Read the model definition and answer for the solid it produces. Units are mm, in the model's axes. Face numbers are marked on the shaded views. A direction names the side the tool comes from. Coordinates: 2 decimals unless noted, no trailing zeros. Loops run counter-clockwise (first coordinate to the right, second up) from the corner with the lowest first, then second, coordinate; pieces in that order, holes last. Notation, with made-up numbers: M -19.5,-22 L 11.5,-22 A10 ccw 11.5,-10 Z; hole C -8.75,13 d8. An arc over 180 degrees is marked long. Use one line per item in the form item = value. Start each with the question number.
1. A tool of negligible diameter and unlimited length cuts with its end or side. For the marked faces 5, 6, 7 and 8, from which of +Z, -Z, +X, -X, +Y, -Y can it reach the whole face along a straight path? Write none if from no direction.
2. Flat-ended cylindrical pins translate along their axes: pin 1 (3.5 mm diameter, centred on x = -19.5, y = -15, fed in from +Z); pin 2 (3.5 mm diameter, centred on x = 17.55, z = 4.4, fed in from +Y); pin 3 (3 mm diameter, centred on y = -28, z = 17.5, fed in from +X). Find the tip coordinate at first contact, or state that the pin passes through.
3. Find the intervals of material crossed by probe 1 along Z at (x, y) = (0, -4) (3 decimals); probe 2 along Z at (x, y) = (0, -25) (3 decimals); probe 3 along Z at (x, y) = (-14, -5), in increasing order. Write a range as [from, to].
4. The part is cut by section B-B (x = 0). Give the vertices of the cut face in (y, z) (3 decimals), plus the area to 3 significant figures.
5. The part is cut by section C-C (z = 3). Give the vertices of the cut face in (x, y).
6. For a pull along Z with two mould halves and no side action, classify the marked faces 1, 2, 3 and 4 as released by +Z, released by -Z, zero draft, split by the parting line, or undercut.
7. The part is cut by section A-A (y = -3). Give the number of separate pieces and of enclosed holes in the cut face, plus the area to 3 significant figures.
from build123d import *

# Parameters (mm, degrees)
F0_R     = 25.85
F0_R_2   = 4.9
F0_R_3   = 2.1
F1_DEPTH = 1.6
F0_R_4   = 27.45
F2_DEPTH = 10
F3_R     = 12.375
F4_DEPTH = 32.5
F6_DEPTH = 5


# Not quite as in the source:
# - ends of sketch curves that miss each other by under 0.0002 mm in the source are joined


with BuildPart() as f1:
    # F0 (on Front) → F1 (new body)
    with BuildSketch(Plane.XZ):
        Circle(F0_R)
        with Locations((0, -3.85)):
            Circle(F0_R_2, mode=Mode.SUBTRACT)
        with Locations((-17.55, 4.4)):
            Circle(F0_R_3, mode=Mode.SUBTRACT)
        with Locations((17.55, 4.4)):
            Circle(F0_R_3, mode=Mode.SUBTRACT)
    extrude(amount=F1_DEPTH)

    # F0 (on Front) → F2 (join)
    with BuildSketch(Plane.XZ):
        Circle(F0_R_4)
        Circle(F0_R, mode=Mode.SUBTRACT)
    extrude(amount=F2_DEPTH)

    # F3 (on face) → F4 (join)
    with BuildSketch(Plane.XZ.offset(1.6)):
        with BuildLine():
            Line((17.55, 9.65), (18.2565056898, 9.65))
            ThreePointArc((18.2565056898, 9.65), (0, 20.65), (-18.2565056898, 9.65))
            Line((-18.2565056898, 9.65), (-17.55, 9.65))
            ThreePointArc((-17.55, 9.65), (-13.8376893988, 8.1123106012), (-12.3, 4.4))
            ThreePointArc((-12.3, 4.4), (-13.8376893988, 0.6876893988), (-17.55, -0.85))
            Line((-17.55, -0.85), (-20.6324986369, -0.85))
            ThreePointArc((-20.6324986369, -0.85), (0, -20.65), (20.6324986369, -0.85))
            Line((20.6324986369, -0.85), (17.55, -0.85))
            ThreePointArc((17.55, -0.85), (12.3, 4.4), (17.55, 9.65))
        make_face()
        with Locations((0, -3.85)):
            Circle(F3_R, mode=Mode.SUBTRACT)
    extrude(amount=F4_DEPTH)

    # F5 (on face) → F6 (join)
    with BuildSketch(Plane.XZ.offset(34.1)):
        with BuildLine():
            ThreePointArc((-17.55, -0.85), (-13.8376893988, 0.6876893988), (-12.3, 4.4))
            ThreePointArc((-12.3, 4.4), (-13.8376893988, 8.1123106012), (-17.55, 9.65))
            ThreePointArc((-17.55, 9.65), (-17.9177743439, 9.6371024462), (-18.2837416824, 9.598473155))
            ThreePointArc((-18.2837416824, 9.598473155), (-20.0300885135, 5.0217580727), (-20.6493606667, 0.1624932498))
            ThreePointArc((-20.6493606667, 0.1624932498), (-19.1802744495, -0.5904614235), (-17.55, -0.85))
        make_face()
        with BuildLine():
            ThreePointArc((-18.2837416824, 9.598473155), (-17.9177743439, 9.6371024462), (-17.55, 9.65))
            Line((-17.55, 9.65), (-18.2565056898, 9.65))
            ThreePointArc((-18.2565056898, 9.65), (-18.2701054669, 9.6242270457), (-18.2837416824, 9.598473155))
        make_face()
        with BuildLine():
            Line((-20.6324986369, -0.85), (-17.55, -0.85))
            ThreePointArc((-17.55, -0.85), (-19.1802744495, -0.5904614235), (-20.6493606667, 0.1624932498))
            ThreePointArc((-20.6493606667, 0.1624932498), (-20.6471369089, -0.3438567505), (-20.6324986369, -0.85))
        make_face()
        with BuildLine():
            ThreePointArc((20.6493606667, 0.1624932498), (20.0300885135, 5.0217580727), (18.2836688601, 9.5984349253))
            ThreePointArc((18.2836688601, 9.5984349253), (17.9177743439, 9.6371024462), (17.55, 9.65))
            ThreePointArc((17.55, 9.65), (12.3, 4.4), (17.55, -0.85))
            ThreePointArc((17.55, -0.85), (19.1802744495, -0.5904614235), (20.6493606667, 0.1624932498))
        make_face()
        with BuildLine():
            Line((17.55, -0.85), (20.6324986369, -0.85))
            ThreePointArc((20.6324986369, -0.85), (20.6456241956, -0.425090078), (20.65, 0))
            ThreePointArc((20.65, 0), (20.6498401661, 0.0812472538), (20.6493606667, 0.1624932498))
            ThreePointArc((20.6493606667, 0.1624932498), (19.1802744495, -0.5904614235), (17.55, -0.85))
        make_face()
        with BuildLine():
            ThreePointArc((18.2836688601, 9.5984349253), (18.2701054669, 9.6242270457), (18.2565056898, 9.65))
            Line((18.2565056898, 9.65), (17.55, 9.65))
            ThreePointArc((17.55, 9.65), (17.9177743439, 9.6371024462), (18.2836688601, 9.5984349253))
        make_face()
    extrude(amount=-F6_DEPTH)


solid = f1.part
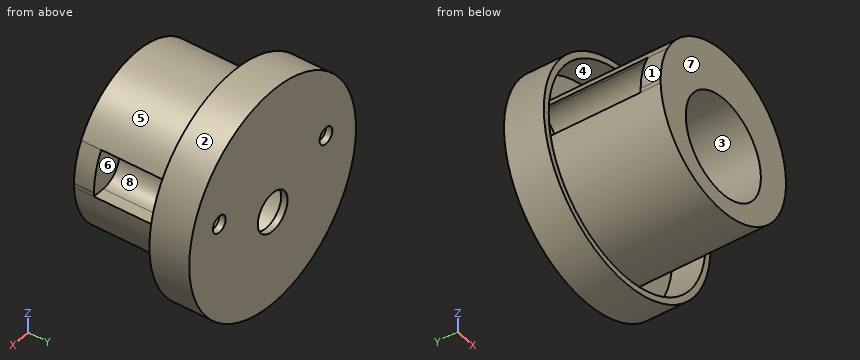
Computed values:
q1.face_5 = -Y
q1.face_6 = +X
q1.face_7 = +Z, -Z, +X, -X, -Y
q1.face_8 = none
q2.pin_1 = 10.55
q2.pin_2 = -29.1
q2.pin_3 = 13.05
q3.probe_1 = [-27.45, -25.85], [-20.65, -16.225], [8.525, 20.65], [25.85, 27.45]
q3.probe_2 = [-20.65, -16.225], [8.525, 20.65]
q3.probe_3 = [-23.61, -21.73], [-15.18, 0.53], [8.27, 15.18], [21.73, 23.61]
q4.outline = M -34.1,-20.65 L -1.6,-20.65 L -1.6,-25.85 L -10,-25.85 L -10,-27.45 L 0,-27.45 L 0,-8.75 L -1.6,-8.75 L -1.6,-16.225 L -34.1,-16.225 Z; M -34.1,8.525 L -1.6,8.525 L -1.6,1.05 L 0,1.05 L 0,27.45 L -10,27.45 L -10,25.85 L -1.6,25.85 L -1.6,20.65 L -34.1,20.65 Z
q4.area = 637 mm²
q5.outline = M -27.29,-10 L -25.68,-10 L -25.68,-1.6 L -19.12,-1.6 L -19.12,0 L -27.29,0 Z; M -20.43,-34.1 L -10.31,-34.1 L -10.31,-1.6 L 10.31,-1.6 L 10.31,-34.1 L 20.43,-34.1 L 20.43,-29.1 L 12.49,-29.1 L 12.49,-1.6 L 15.98,-1.6 L 15.98,0 L -15.98,0 L -15.98,-1.6 L -12.49,-1.6 L -12.49,-29.1 L -20.43,-29.1 Z; M 19.12,-1.6 L 25.68,-1.6 L 25.68,-10 L 27.29,-10 L 27.29,0 L 19.12,0 Z
q6.face_1 = released by +Z
q6.face_2 = split by the parting line
q6.face_3 = undercut
q6.face_4 = undercut
q7.separate_pieces = 2
q7.enclosed_holes = 2
q7.area = 990 mm²
